Source: three-view drawing plus pictorial views. Frame: mm from the lowest corner of the part. Give positions to 0.01 mm unless a question says otherwise; leave off trailing zeros. Loops run counter-clockwise (first coordinate to the right, second up) from the corner with the lowest first, then second, coordinate; pieces in that order, holes last. Notation, with made-up numbers: (-25.5, 45) - (24.5, 45) arc R35 ccw to (24.5, 80) - close; hole circle Ø11 at (50.25, 11.5). An arc over 180 degrees is marked (long way). One line per item, written item: value.
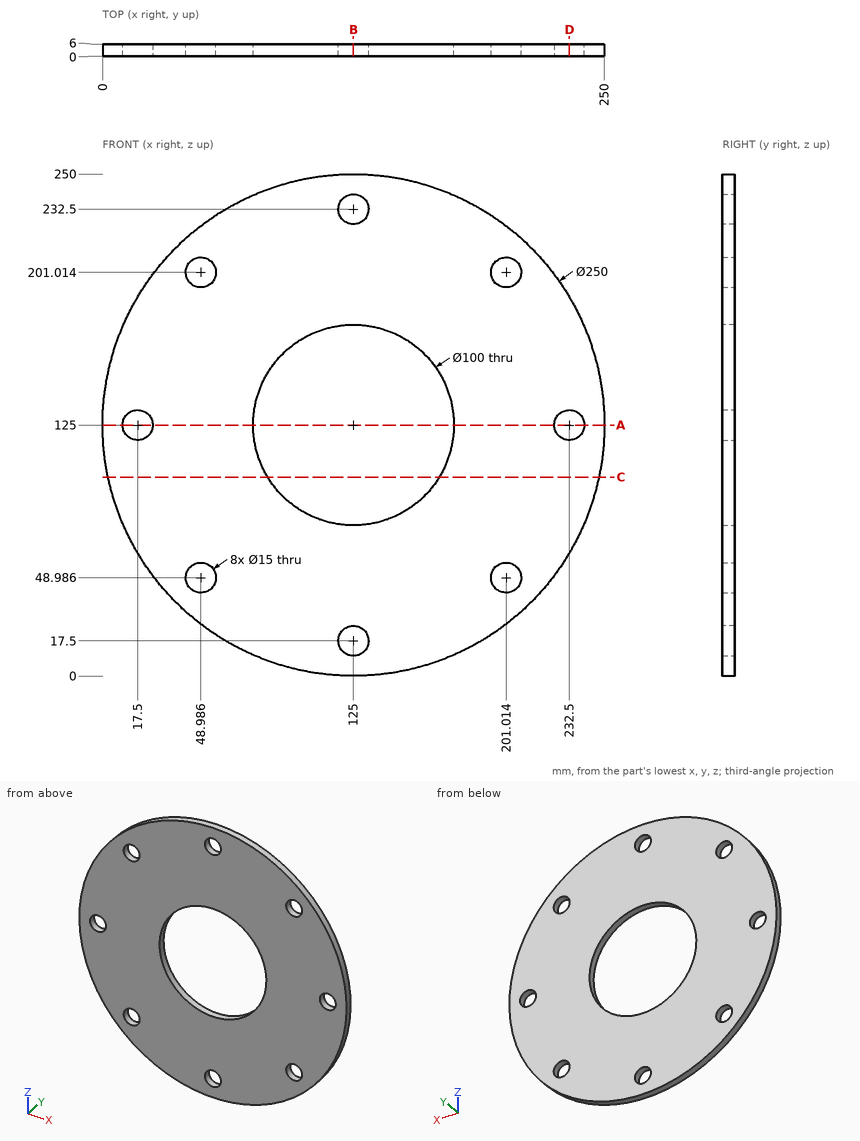
Item 1: Section A-A, the plane z = 125. Output: boundary loops of the cut face in (x, y), and give its area (3 significant figures).
Verdict:
outline: (0, 0) - (10, 0) - (10, 6) - (0, 6) - close; (25, 0) - (75, 0) - (75, 6) - (25, 6) - close; (175, 0) - (225, 0) - (225, 6) - (175, 6) - close; (240, 0) - (250, 0) - (250, 6) - (240, 6) - close
area: 720 mm^2
Item 2: Section D-D, the plane x = 232.5. Output: boundary loops of the cut face in (y, z).
Verdict:
outline: (0, 61.21) - (6, 61.21) - (6, 117.5) - (0, 117.5) - close; (0, 132.5) - (6, 132.5) - (6, 188.79) - (0, 188.79) - close
Item 3: Section B-B, the plane x = 125. Output: boundary loops of the cut face in (y, z), and give its area (3 significant figures).
Verdict:
outline: (0, 0) - (6, 0) - (6, 10) - (0, 10) - close; (0, 25) - (6, 25) - (6, 75) - (0, 75) - close; (0, 175) - (6, 175) - (6, 225) - (0, 225) - close; (0, 240) - (6, 240) - (6, 250) - (0, 250) - close
area: 720 mm^2
Item 4: Material intervals for L1, parallel to Z at x = 125.5, y = 1.9; L2, parallel to Z at x = 124, y = 0.9; L3, parallel to Z at x = 200, y = 2.1, sorted ascending.
Verdict:
L1: z = 0 to 10.02, 24.98 to 75, 175 to 225.02, 239.98 to 250
L2: z = 0 to 10.07, 24.93 to 75.01, 174.99 to 225.07, 239.93 to 250
L3: z = 25 to 41.55, 56.42 to 193.58, 208.45 to 225
Item 5: Pin query (flat end, axial travel): P1, Ø1, axis at x = 151.5, y = 2.5, coming from the -Z side; P2, Ø2, axis at x = 101.5, y = 0.5, coming from the +Z side; P3, Ø1, axis at y = 5.5, z = 44.5, coming from the +X side. Return the tip coordinate at first contact, or that it passes through.
Verdict:
P1: stops at z = 2.73
P2: stops at z = 247.96
P3: stops at x = 221.05
Item 6: Section C-C, the plane z = 99. Output: boundary loops of the cut face in (x, y).
Verdict:
outline: (2.73, 0) - (82.29, 0) - (82.29, 6) - (2.73, 6) - close; (167.71, 0) - (247.27, 0) - (247.27, 6) - (167.71, 6) - close
